```python
from build123d import *

# Parameters (mm, degrees)
BOSS_EXTRUDE1_DEPTH        = 50.8
SKETCH5_W                  = 15.875
SKETCH5_H                  = 50.8
BOSS_EXTRUDE2_DEPTH        = 19.05
F_4_40_TAPPED_HOLE1_REACH  = 64.104
F_4_40_TAPPED_HOLE1_BORE_R = 1.1303
SKETCH9_W                  = 32.004
SKETCH9_H                  = 50.8
BOSS_EXTRUDE4_DEPTH        = 203.2


with BuildPart() as part:
    # Sketch2 → Boss-Extrude1 (new body)
    with BuildSketch(Plane(origin=(0, 0, 0), x_dir=(1, 0, 0), z_dir=(0, 1, 0))):
        Polygon((0, 0), (0, 15.875), (3.175, 15.875), (3.175, 3.175), (9.779, 3.175), (9.779, 15.875), (12.954, 15.875), (12.954, 0), align=None)
    extrude(amount=BOSS_EXTRUDE1_DEPTH)

    # Sketch5 → Boss-Extrude2 (add)
    with BuildSketch(Plane(origin=(12.954, 0, 0), x_dir=(0, 0, -1), z_dir=(1, 0, 0))):
        with Locations((7.9375, 25.4)):
            Rectangle(SKETCH5_W, SKETCH5_H)
    extrude(amount=BOSS_EXTRUDE2_DEPTH)

    # #4-40 Tapped Hole1 bore → #4-40 Tapped Hole1 (cut, up to next)
    with BuildSketch(Plane(origin=(32.004, 0, 0), x_dir=(0, 0, -1), z_dir=(1, 0, 0)), mode=Mode.PRIVATE) as f_4_40_tapped_hole1_sk1:
        with Locations((7.9375, 12.7)):
            Circle(F_4_40_TAPPED_HOLE1_BORE_R)
    f_4_40_tapped_hole1_tool1 = extrude(f_4_40_tapped_hole1_sk1.sketch, amount=-F_4_40_TAPPED_HOLE1_REACH, mode=Mode.PRIVATE) & part.part
    # #4-40 Tapped Hole1 bore → #4-40 Tapped Hole1 (cut, up to next)
    with BuildSketch(Plane(origin=(32.004, 0, 0), x_dir=(0, 0, -1), z_dir=(1, 0, 0)), mode=Mode.PRIVATE) as f_4_40_tapped_hole1_sk2:
        with Locations((7.9375, 38.1)):
            Circle(F_4_40_TAPPED_HOLE1_BORE_R)
    f_4_40_tapped_hole1_tool2 = extrude(f_4_40_tapped_hole1_sk2.sketch, amount=-F_4_40_TAPPED_HOLE1_REACH, mode=Mode.PRIVATE) & part.part
    add(f_4_40_tapped_hole1_tool1.solids().sort_by_distance((32.004, 12.7, -7.9375))[0], mode=Mode.SUBTRACT)
    add(f_4_40_tapped_hole1_tool2.solids().sort_by_distance((32.004, 38.1, -7.9375))[0], mode=Mode.SUBTRACT)

    # Sketch9 → Boss-Extrude4 (add)
    with BuildSketch(Plane.XY):
        with Locations((16.002, 25.4)):
            Rectangle(SKETCH9_W, SKETCH9_H)
    extrude(amount=BOSS_EXTRUDE4_DEPTH)


solid = part.part
```
Here's how the part is built. I have some questions about the finished solid (model axes, mm). A direction names the side the tool comes from. Round coordinates to 2 decimals unless told otherwise and drop trailing zeros. Loops run counter-clockwise (first coordinate to the right, second up) from the corner with the lowest first, then second, coordinate; pieces in that order, holes last. Notation, with made-up numbers: (44, 33.25) -> (87, 33.25) arc R14 ccw to (87, 47.25) -> close; hole circle Ø5 at (-27, 35). An arc over 180 degrees is marked (long way). Answer as CSV lines item,"result". Start each with the question number.
1. I need wall thicknesses on probe 1 along Z at (x, y) = (23, 38) (3 decimals); probe 2 along Z at (x, y) = (4, 9.5) (3 decimals). Which ranges of each line are inside material? Lowest first, please. Write a range as from..to.
2. For faces 5 (the face through (3.175, 25, -10)), 6 (the face through (16, 50.8, 92)), which set-ups out of +Z, -Z, +X, -X, +Y, -Y let a thin tool reach every point of the face, with its end or its side?
3. If we mould it in two halves opening along X, with no side actions, what happens to faces 1 (the face through (32.004, 25, 92)), 2 (the face through (6, 25, -3.175)), 3 (the face through (0, 25, 92)), 4 (the face through (21, 25, -15.875))? For each: pulls with the +X half, pulls with the -X half, needs draft (parallel to the pull), parting line crosses it, or undercut.
4. I'm going to push a flat-ended pin straight in: P1, Ø3, axis at x = 6, y = 36.5, coming from the -Z side (3 decimals). Where does the tip first touch, or does it pass through?
5. Imagine slicing it at A-A on x = 5. Write out the boundary of the cut face in (y, z) (3 decimals), plus the area to 3 significant figures.
Solution:
1,probe 1,"-15.875..-9.063, -6.812..203.2"
1,probe 2,"-3.175..203.2"
2,face 5,"-Z, +Y, -Y"
2,face 6,"+Z, -Z, +X, -X, +Y"
3,face 1,"pulls with the +X half"
3,face 2,"undercut"
3,face 3,"pulls with the -X half"
3,face 4,"needs draft"
4,P1,"z = -3.175"
5,outline,"(0, -3.175) -> (50.8, -3.175) -> (50.8, 203.2) -> (0, 203.2) -> close"
5,area,"10,500 mm²"
